Source: CAD feature listing. Evaluate the final solid. Frame: model axes, mm. A direction names the side the tool comes from. Coordinates: 2 decimals unless noted, no trailing zeros. Loops run counter-clockwise (first coordinate to the right, second up) from the corner with the lowest first, then second, coordinate; pieces in that order, holes last. Notation, with made-up numbers: (11.25, -20) -> (56.25, -20) arc R26 ccw to (56.25, 16) -> close; hole circle Ø10 at (6, 35). An arc over 180 degrees is marked (long way). Answer as a JSON object with one key per item and string values. Group by question number.
from build123d import *

# Parameters (mm, degrees)
SKETCH2_R                                         = 45
SKETCH2_R_2                                       = 14.4
BOSS_EXTRUDE1_DEPTH                               = 28
CSK_FOR_M2_FLAT_HEAD_MACHINE_SCREW2_D             = 2.2
CSK_FOR_M2_FLAT_HEAD_MACHINE_SCREW2_DEPTH         = 60.2
CSK_FOR_M2_FLAT_HEAD_MACHINE_SCREW2_CSINK_D       = 4.4
CSK_FOR_M2_FLAT_HEAD_MACHINE_SCREW2_CSINK_ANGLE   = 90
CSK_FOR_M2_FLAT_HEAD_MACHINE_SCREW2_TIP           = 0.660946681
CSK_FOR_0_FLAT_HEAD_MACHINE_SCREW_100_D           = 1.778
CSK_FOR_0_FLAT_HEAD_MACHINE_SCREW_100_DEPTH       = 60.2
CSK_FOR_0_FLAT_HEAD_MACHINE_SCREW_100_CSINK_D     = 3.0226
CSK_FOR_0_FLAT_HEAD_MACHINE_SCREW_100_CSINK_ANGLE = 100
CSK_FOR_0_FLAT_HEAD_MACHINE_SCREW_100_TIP         = 0.53416509


with BuildPart() as part:
    # Sketch2 → Boss-Extrude1 (new body)
    with BuildSketch(Plane.XY):
        Circle(SKETCH2_R)
        Circle(SKETCH2_R_2, mode=Mode.SUBTRACT)
    extrude(amount=BOSS_EXTRUDE1_DEPTH)

    # CSK for M2 Flat Head Machine Screw2
    with Locations(Plane(origin=(44.500938933, 6.683295151, 12.740574547), x_dir=(-0.148517670011, 0.98890975407, 0), z_dir=(0.98890975407, 0.148517670011, 0))):
        with Locations((-1e-09, 0)):
            CounterSinkHole(CSK_FOR_M2_FLAT_HEAD_MACHINE_SCREW2_D / 2, CSK_FOR_M2_FLAT_HEAD_MACHINE_SCREW2_CSINK_D / 2, depth=CSK_FOR_M2_FLAT_HEAD_MACHINE_SCREW2_DEPTH, counter_sink_angle=CSK_FOR_M2_FLAT_HEAD_MACHINE_SCREW2_CSINK_ANGLE)
            with Locations((0, 0, -(CSK_FOR_M2_FLAT_HEAD_MACHINE_SCREW2_DEPTH + CSK_FOR_M2_FLAT_HEAD_MACHINE_SCREW2_TIP / 2))):  # 118° drill point
                Cone(0, CSK_FOR_M2_FLAT_HEAD_MACHINE_SCREW2_D / 2, CSK_FOR_M2_FLAT_HEAD_MACHINE_SCREW2_TIP, mode=Mode.SUBTRACT)

    # CSK for #0 Flat Head Machine Screw (100)1
    with Locations(Plane(origin=(-19.959479504, 40.331367172, 13.936569292), x_dir=(0.896252603816, 0.443543988972, 0), z_dir=(-0.443543988972, 0.896252603816, 0))):
        with Locations((0, 0)):
            CounterSinkHole(CSK_FOR_0_FLAT_HEAD_MACHINE_SCREW_100_D / 2, CSK_FOR_0_FLAT_HEAD_MACHINE_SCREW_100_CSINK_D / 2, depth=CSK_FOR_0_FLAT_HEAD_MACHINE_SCREW_100_DEPTH, counter_sink_angle=CSK_FOR_0_FLAT_HEAD_MACHINE_SCREW_100_CSINK_ANGLE)
            with Locations((0, 0, -(CSK_FOR_0_FLAT_HEAD_MACHINE_SCREW_100_DEPTH + CSK_FOR_0_FLAT_HEAD_MACHINE_SCREW_100_TIP / 2))):  # 118° drill point
                Cone(0, CSK_FOR_0_FLAT_HEAD_MACHINE_SCREW_100_D / 2, CSK_FOR_0_FLAT_HEAD_MACHINE_SCREW_100_TIP, mode=Mode.SUBTRACT)


solid = part.part
1. Section query A-A on y = 0. Return loops of the section in (x, z), then the cut area to 3 significant figures.
2. Mould query, pull axis X, two halves, no side actions, for faces 3 (the face through (-1.87, 14.28, 13.8)), 4 (the face through (-11, 11, 28)), 5 (the face through (20.765, -39.923, 13.804)), 6 (the face through (-13.694, 25.819, 14.277)). Classes: pulls with the +X half, pulls with the -X half, needs draft (parallel to the pull), parting line crosses it, or undercut.
3. Reachability of faces 1 (the face through (-15.549, -2.488, 12.624)), 2 (the face through (-11, 11, 0)) from +Z, -Z, +X, -X, +Y, -Y: full face, straight path, thin tool, end or side. Return the list, or none.
4. Ray query, L1, parallel to Y at x = 0, z = 9.5; L2, parallel to X at y = 30, z = 14.25; L3, parallel to X at y = 29, z = 12. Return the intervals inside material, ascending.
5. Pin query (flat end, axial travel): pin 1 Ø4 at (y, z) = (32.5, 13.5) entering from -X; pin 2 Ø10 at (x, z) = (30.5, 18.5) entering from -Y; pin 3 Ø1.5 at (x, z) = (-10, 6.5) entering from +Y. Return the tip coordinate at first contact, or that it passes through.
6. Section query C-C on z = 21.5. Return loops of the section in (x, y).
7. Section query D-D on x = -36. Return loops of the section in (y, z).
Solved:
{
 "1": {"outline": "(-45, 0) -> (-14.4, 0) -> (-14.4, 28) -> (-45, 28) -> close; (14.4, 0) -> (45, 0) -> (45, 28) -> (14.4, 28) -> close", "area": "1,710 mm^2"},
 "2": {"face 3": "undercut", "face 4": "needs draft", "face 5": "parting line crosses it", "face 6": "undercut"},
 "3": {"face 1": "none", "face 2": "-Z, +X, -X, +Y, -Y"},
 "4": {"L1": "-45 to -14.4, 14.4 to 45", "L2": "-33.54 to -15.77, -13.92 to 33.54", "L3": "-34.41 to 34.41"},
 "5": {"pin 1": "x = -33.09", "pin 2": "y = -37.08", "pin 3": "y = 44.04"},
 "6": {"outline": "circle Ø90 at (0, 0); hole circle Ø28.8 at (0, 0)"},
 "7": {"outline": "(-27, 0) -> (27, 0) -> (27, 28) -> (-27, 28) -> close"}
}
